For this review, take the finished solid that the model builds, in its own axes (mm). A direction names the side the tool comes from. Coordinates: 2 decimals unless noted, no trailing zeros. Loops run counter-clockwise (first coordinate to the right, second up) from the corner with the lowest first, then second, coordinate; pieces in that order, holes last. Notation, with made-up numbers: (27.25, 13) - (55.25, 13) arc R20 ccw to (55.25, 46) - close; hole circle Ø7 at (15, 51). An arc over 180 degrees is marked (long way). One line per item, written item: value. Start each with the question number.
1. The part is to be moulded in two halves that separate along X. For faces 1 (the face through (0, 3, 53)), 2 (the face through (0, 2.769, 55)), 3 (the face through (-2.17, -9.76, 1.48)), 4 (the face through (0, 0, 0)), say which applies: released by +X, released by -X, zero draft, split by the parting line, or undercut.
2. For faces 5 (the face through (0, 0, 58)), 6 (the face through (0.543, 3, 55)), 7 (the face through (-0.1, -4.3, 3)), list the 3-axis set-ups (+Z, -Z, +X, -X, +Y, -Y) from which the entire face can be reached by the end or side of a thin tool; tool diameter is ignored.
3. Take a section at B-B, the plane x = -3. State the section outline as (y, z) points, and give its area (3 significant figures).
4. To check wall thickness, follow line 1 (Z direction, x = -1.25, y = 7.25); line 2 (Y direction, x = 0, z = 55.5); line 3 (X direction, y = 0, z = 27). State the ranges of each line that lie inside material, in increasing order. Write a range as from..to.
5. Take a section at C-C, the plane z = 31. State the section outline as (x, y) points.
6. Take a section at D-D, the plane x = -5.5. State the section outline as (y, z) points.
7. Insertion check: pin 1 (3 mm diameter, centred on x = 5, z = 35, fed in from -Y); pin 2 (1 mm diameter, centred on x = 2.5, y = 4.5, fed in from +Z); pin 3 (5 mm diameter, centred on x = -4.5, z = 51, fed in from -Y); pin 4 (12 mm diameter, centred on x = -5, y = -2, fed in from -Z). Each pin has a flat end and moves straight along its axis. Give the tip position at first contact, or say it passes through.
8. Take a section at A-A, the plane y = 0. State the section outline as (x, z) points, and give its area (3 significant figures).
```python
from build123d import *

# Parameters (mm, degrees)
SKETCH1_R           = 10
BOSS_EXTRUDE1_DEPTH = 3
SKETCH2_R           = 4
BOSS_EXTRUDE2_DEPTH = 55
CUT_EXTRUDE1_DEPTH  = 10


with BuildPart() as part:
    # Sketch1 → Boss-Extrude1 (new body)
    with BuildSketch(Plane.XY):
        Circle(SKETCH1_R)
    extrude(amount=BOSS_EXTRUDE1_DEPTH)

    # Sketch2 → Boss-Extrude2 (add)
    with BuildSketch(Plane.XY.offset(3)):
        Circle(SKETCH2_R)
    extrude(amount=BOSS_EXTRUDE2_DEPTH)

    # Sketch3 → Cut-Extrude1 (cut)
    with BuildSketch(Plane.XY.offset(53)):
        with BuildLine():
            Line((-0.5, 3.968626967), (-0.5, 2.768626967))
            Line((-0.5, 2.768626967), (0.543300129, 2.768626967))
            Line((0.543300129, 2.768626967), (0.543300129, 3.962931361))
            ThreePointArc((0.543300129, 3.962931361), (0.021836558, 3.999940395), (-0.5, 3.968626967))
        make_face()
    extrude(amount=CUT_EXTRUDE1_DEPTH, mode=Mode.SUBTRACT)


solid = part.part
```
Solutions:
1. face 1: undercut
1. face 2: undercut
1. face 3: split by the parting line
1. face 4: zero draft
2. face 5: +Z, +X, -X, +Y, -Y
2. face 6: +Z, +Y
2. face 7: +Z
3. outline: (-9.54, 0) - (9.54, 0) - (9.54, 3) - (2.65, 3) - (2.65, 58) - (-2.65, 58) - (-2.65, 3) - (-9.54, 3) - close
3. area: 348 mm2
4. line 1: 0..3
4. line 2: -4..2.77
4. line 3: -4..4
5. outline: circle Ø8 at (0, 0)
6. outline: (-8.35, 0) - (8.35, 0) - (8.35, 3) - (-8.35, 3) - close
7. pin 1: y = -1.94
7. pin 2: z = 3
7. pin 3: y = -3.46
7. pin 4: z = 0
8. outline: (-10, 0) - (10, 0) - (10, 3) - (4, 3) - (4, 58) - (-4, 58) - (-4, 3) - (-10, 3) - close
8. area: 500 mm2
